Source: CAD feature listing. Evaluate the final solid. Frame: model axes, mm. Give positions to 0.01 mm unless a question says otherwise; leave off trailing zeros. Loops run counter-clockwise (first coordinate to the right, second up) from the corner with the lowest first, then second, coordinate; pieces in that order, holes last.
```python
from build123d import *

# Parameters (mm, degrees)
F0_R     = 12.7
F1_DEPTH = 3.175
F2_R     = 3.302
F3_DEPTH = 25.4
F4_R     = 3.831574
F5_DEPTH = 25.4


with BuildPart() as f1:
    # F0 (on Top) → F1 (new body)
    with BuildSketch(Plane.XY):
        Circle(F0_R)
    extrude(amount=F1_DEPTH)

    # F2 (on Top) → F3 (cut)
    with BuildSketch(Plane.XY):
        Circle(F2_R)
    extrude(amount=F3_DEPTH, mode=Mode.SUBTRACT)

    # F4 (on Top) → F5 (cut)
    with BuildSketch(Plane.XY):
        with Locations((0, 8.084333)):
            Circle(F4_R)
        with Locations((-8.084333, 0)):
            Circle(F4_R)
        with Locations((0, -8.084333)):
            Circle(F4_R)
        with Locations((8.084333, 0)):
            Circle(F4_R)
    extrude(amount=F5_DEPTH, mode=Mode.SUBTRACT)


solid = f1.part
```
(1) Section A-A, the plane x = 0. Return the cut outline in (y, z) (3 decimals).
A:
outline: (-12.7, 0) - (-11.916, 0) - (-11.916, 3.175) - (-12.7, 3.175) - close; (-4.253, 0) - (-3.302, 0) - (-3.302, 3.175) - (-4.253, 3.175) - close; (3.302, 0) - (4.253, 0) - (4.253, 3.175) - (3.302, 3.175) - close; (11.916, 0) - (12.7, 0) - (12.7, 3.175) - (11.916, 3.175) - close
(2) Mould query, pull axis Y, two halves, no side actions, for faces 1 (the cylindrical face through (-0.499, 11.883, 1.565)), 2 (the cylindrical face through (-2.75, -12.4, 1.57)), 3 (the flat face through (3, -3, 3.175)). Classes: pulls with the +Y half, pulls with the -Y half, needs draft (parallel to the pull), parting line crosses it, or undercut.
A:
face 1: undercut
face 2: parting line crosses it
face 3: needs draft
(3) Section B-B, the plane y = 4.75. Return the cut outline in (x, z) (3 decimals).
A:
outline: (-11.778, 0) - (-1.888, 0) - (-1.888, 3.175) - (-11.778, 3.175) - close; (1.888, 0) - (11.778, 0) - (11.778, 3.175) - (1.888, 3.175) - close
(4) Section D-D, the plane x = -5.75. Return the cut outline in (y, z) (3 decimals), then the cut area to 3 significant figures.
A:
outline: (-11.324, 0) - (-3.038, 0) - (-3.038, 3.175) - (-11.324, 3.175) - close; (3.038, 0) - (11.324, 0) - (11.324, 3.175) - (3.038, 3.175) - close
area: 52.6 mm2
(5) First-contact query: pin 1 (6 mm diameter, centred on x = 8.08, y = 0, fed in from +Z). Flat tip, straight axial feed; report the tip coordinate or a pass-through.
A:
pin 1: passes through
(6) Ray query, line 1 along Y through (x, z) = (0, 2.4); line 2 along Y through (x, z) = (1, 2.95); line 3 along X through (y, z) = (0.5, 2.1). Return the intervals inside material, ascending.
A:
line 1: y = -12.7 to -11.92, -4.25 to -3.3, 3.3 to 4.25, 11.92 to 12.7
line 2: y = -12.66 to -11.78, -4.39 to -3.15, 3.15 to 4.39, 11.78 to 12.66
line 3: x = -12.69 to -11.88, -4.29 to -3.26, 3.26 to 4.29, 11.88 to 12.69
